Autodesk Inventor part; units mm, degrees
ref_plane "YZ Plane" through (0, 0, 0) normal (1, 0, 0) x (0, 1, 0)
ref_plane "XZ Plane" through (0, 0, 0) normal (0, 1, 0) x (-1, 0, 0)
ref_plane "XY Plane" through (0, 0, 0) normal (0, 0, 1) x (1, 0, 0)
sketch "Sketch1" plane through (0, 0, 0) normal (0, 0, 1) x (1, 0, 0)
  circle A0 centre (0, 0) radius 1.5
  circle A1 centre (0, 0) radius 3.75
  circle A2 centre (0, 0) radius 6 construction
  line L0 (0, 0) -> (0, 6) construction
  circle A3 centre (-0.25, 10.7596) radius 4.7625
  line L1 (0, 0) -> (0, 6) construction
  line L2 (3.75, 0) -> (3.75, 6)
  line L3 (-3.75, 6) -> (-3.75, 0)
  arc A4 (-3.75, 0) -> (3.75, 0) centre (0, 0) ccw
  arc A5 (3.75, 6) -> (-2.25, 3) centre (0, 6) ccw
  arc A6 (-3.6447, 0.8824) -> (-3.6447, 5.1176) centre (-12.392, 3) ccw
  point P0 (0, 3)
  point P1 (-3.6798, 6.7221)
  point P2 (3.75, 0)
  point P3 (3.3637, 7.6576)
  point P4 (-3.75, 0)
  point P5 (-3.5189, 7.2961)
  dimension "d2" = 12
  dimension "d0" = 3
  dimension "d1" = 7.5
  dimension "d3" = 9.525
  dimension "d4" = 3.75
  dimension "d9" = 0.25
  dimension "d10" = 9
extrude "Extrusion1" add sketch "Sketch1" along normal blind 4.7625 contours A1 | A1 A5 A3 L2 | A1 A6 A5 | L3 A5 A6 A1
fillet "Fillet1" radius 1.5 2 edges at (3.3637, 7.6576, 2.3813) (-3.5189, 7.2961, 2.3813)
sketch "Sketch2" plane through (0, 0, 0) normal (0, 0, -1) x (-1, 0, 0)
  line L0 (-3.75, 0) -> (-3.75, 5.0177)
  arc A0 (-3.75, 0) -> (3.75, 0) centre (0, 0) ccw
  circle A1 centre (0, 0) radius 1.5
  circle A2 centre (0, 0) radius 6.9991 construction
  arc A3 (3.75, 4.825) -> (1.771, 6.2465) centre (2.25, 4.825) ccw
  arc A4 (-1.6512, 6.393) -> (1.771, 6.2465) centre (0.25, 10.7596) ccw
  arc A5 (-1.6512, 6.393) -> (-3.75, 5.0177) centre (-2.25, 5.0177) ccw
  line L1 (3.75, 4.825) -> (3.75, 0)
  arc A6 (-1.6512, 6.393) -> (-3.75, 5.0177) centre (-2.25, 5.0177) ccw
equation "\"d4\" = 0.5 * d1"
properties part number "Cam - Lever" material "Nylon 6/6"
Source: CAD feature listing. Evaluate the final solid. Frame: model axes, mm. Coordinates: 2 decimals unless noted, no trailing zeros. Loops run counter-clockwise (first coordinate to the right, second up) from the corner with the lowest first, then second, coordinate; pieces in that order, holes last. Notation, with made-up numbers: M 87.25,-23 L 112.25,-23 A11 ccw 112.25,-19 Z; hole C 46,11 d5. An arc over 180 degrees is marked long. Put each result on its own line as item: value. Start each with the question number.
1) Cut plane B-B on y = 0.5. Return the cut outline in (x, z), then the cut area to 3 significant figures.
2) Pull-direction query (Y, two-part tool) for faces 1 (the face through (0, 3, 4.762)), 2 (the face through (0.08, -3.75, 2.35)), 3 (the face through (-1.5, -0.07, 2.35)); classes: pulls with the +Y half, pulls with the -Y half, needs draft (parallel to the pull), parting line crosses it, or undercut.
3) Contact query for flat-ended pins moving along their axis: pin 1 Ø1 at (y, z) = (-1.5, 1) entering from -X; pin 2 Ø2 at (x, z) = (-1.5, 3) entering from +Y. Output: stop coordinate, or through.
4) Cut plane A-A on x = 0. Return the cut outline in (y, z), then the cut area to 3 significant figures.
5) Ray query, L1, parallel to Y at x = 0, z = 2.55; L2, parallel to X at y = -0.25, z = 2.3; L3, parallel to X at y = -0.75, z = 3.8. Return the intervals inside material, ascending. Write a range as from..to.
The answers:
1. outline: M -3.75,0 L -1.41,0 L -1.41,4.76 L -3.75,4.76 Z; M 1.41,0 L 3.75,0 L 3.75,4.76 L 1.41,4.76 Z
1. area: 22.2 mm²
2. face 1: needs draft
2. face 2: pulls with the -Y half
2. face 3: undercut
3. pin 1: stops at x = -3.61
3. pin 2: stops at y = 6.33
4. outline: M -3.75,0 L -1.5,0 L -1.5,4.76 L -3.75,4.76 Z; M 1.5,0 L 6,0 L 6,4.76 L 1.5,4.76 Z
4. area: 32.2 mm²
5. L1: y = -3.75..-1.5, 1.5..6
5. L2: x = -3.74..-1.48, 1.48..3.74
5. L3: x = -3.67..-1.3, 1.3..3.67
